Work out the finished part from the listing and answer in its coordinate system (mm). Face numbers are marked on the shaded views. A direction names the side the tool comes from. Give positions to 0.01 mm unless a question says otherwise; leave off trailing zeros. Order: outer loops, then holes, each group sorted by start corner. A loop starts at its lowest first (then second) coordinate and runs counter-clockwise, first axis right, second up. Notation, with made-up numbers: (-12, 62.25) - (33, 62.25) arc R20 ccw to (33, 90.25) - close; hole circle Ø11 at (10.5, 1). An arc over 180 degrees is marked (long way). Return JSON: item names as keys, results as strings. Group by question number.
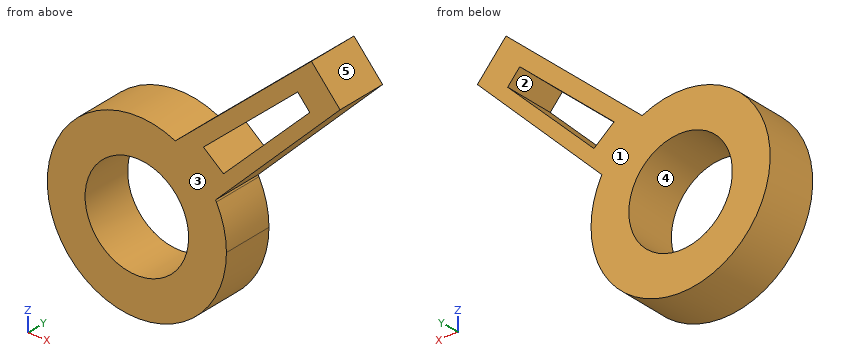
from build123d import *

# Parameters (mm, degrees)
F0_R     = 9.101215
F1_DEPTH = 9.144
F3_DEPTH = 9.144


with BuildPart() as f1:
    # F0 (on Front) → F1 (new body)
    with BuildSketch(Plane.XZ):
        with BuildLine():
            ThreePointArc((-19.067402, -17.204188), (-40.212946, -39.010997), (-10.913195, -30.998787))
            ThreePointArc((-10.913195, -30.998787), (-11.36082, -27.271094), (-12.678245, -23.755351))
            ThreePointArc((-12.678245, -23.755351), (-15.386403, -20.005377), (-19.067402, -17.204188))
        make_face()
        with Locations((-26.658566, -30.998787)):
            Circle(F0_R, mode=Mode.SUBTRACT)
    extrude(amount=F1_DEPTH)

    # F2 (on Front) → F3 (join)
    with BuildSketch(Plane.XZ):
        Polygon((4.029281, 4.029281), (-22.448849, -18.995181), (-14.390289, -25.039099), (9.060461, -1.756575), align=None)
        Polygon((-11.423091, -18.922271), (-14.96415, -16.013544), (1.608393, -1.602637), (3.734771, -4.047971), align=None, mode=Mode.SUBTRACT)
    extrude(amount=F3_DEPTH)


solid = f1.part
1. Consider probe 1 along Z at (x, y) = (-1.5, -7.5); probe 2 along X at (y, z) = (-4.75, -29); probe 3 along X at (y, z) = (-2.5, -29.5). Determine where each line is inside the solid, lowest interval first. Write a range as from..to.
2. A tool of negligible diameter and unlimited length cuts with its end or side. For the marked faces 1 and 2, from which of +Z, -Z, +X, -X, +Y, -Y can it reach the whole face along a straight path? Write none if from no direction.
3. Determine the mould class of the marked faces 3, 4 and 5 for opening direction X: released by +X, released by -X, zero draft, split by the parting line, or undercut.
4. The part is cut by section D-D (x = -37). Give the vertices of the cut face in (y, z), and give its area (3 significant figures).
5. Each of these flat-tipped pins is pushed along its axis until it touches: pin 1 (4 mm diameter, centred on x = -28, y = -7, fed in from -Z); pin 2 (14.5 mm diameter, centred on x = -26.66, z = -31, fed in from +Y); pin 3 (1 mm diameter, centred on x = -20.5, y = -5, fed in from -Z); pin 4 (3 mm diameter, centred on y = -6, z = -33, fed in from +X). Where does it stop, or does it pass through?
6. The part is cut by section C-C (z = -12). Give the vertices of the cut face in (x, y), and give its area (3 significant figures).
7. The part is cut by section A-A (y = -3.25). Give the vertices of the cut face in (x, z), and give its area (3 significant figures).
8. The part is cut by section B-B (x = -27). Give the vertices of the cut face in (y, z).
Answers:
{
 "1": {"probe 1": "z = -12.24..-9.18, -4.31..-0.78", "probe 2": "x = -42.28..-35.54, -17.78..-11.04", "probe 3": "x = -42.33..-35.64, -17.68..-10.98"},
 "2": {"face 1": "+Z, -Z, +X, -X, +Y", "face 2": "+Y, -Y"},
 "3": {"face 3": "zero draft", "face 4": "undercut", "face 5": "released by +X"},
 "4": {"outline": "(-9.14, -42.87) - (0, -42.87) - (0, -19.13) - (-9.14, -19.13) - close", "area": "217 mm^2"},
 "5": {"pin 1": "stops at z = -46.74", "pin 2": "passes through", "pin 3": "stops at z = -45.69", "pin 4": "stops at x = -10.92"},
 "6": {"outline": "(-14.4, -9.14) - (-10.35, -9.14) - (-10.35, 0) - (-14.4, 0) - close; (-4.37, -9.14) - (-1.26, -9.14) - (-1.26, 0) - (-4.37, 0) - close", "area": "65.5 mm^2"},
 "7": {"outline": "(-19.9, -16.78) arc R15.75 ccw (long way) to (-10.91, -31) arc R15.75 ccw to (-12.68, -23.76) arc R15.75 ccw to (-12.82, -23.48) - (9.06, -1.76) - (4.03, 4.03) - close; hole circle Ø18.2 at (-26.66, -31); hole (-14.96, -16.01) - (-11.42, -18.92) - (3.73, -4.05) - (1.61, -1.6) - close", "area": "701 mm^2"},
 "8": {"outline": "(-9.14, -46.74) - (0, -46.74) - (0, -40.09) - (-9.14, -40.09) - close; (-9.14, -21.9) - (0, -21.9) - (0, -15.26) - (-9.14, -15.26) - close"}
}
